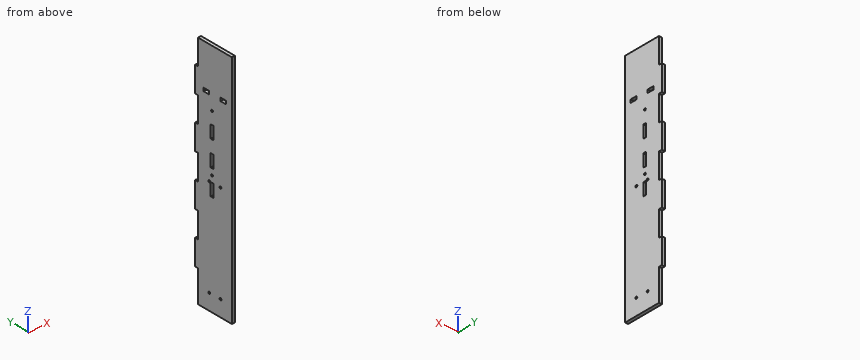
```python
from build123d import *

# Parameters (mm, degrees)
SKETCH1_W           = 6.35
SKETCH1_H           = 76.2
BOSS_EXTRUDE1_DEPTH = 457.2
SKETCH2_W           = 6.35
SKETCH2_H           = 50.8
BOSS_EXTRUDE2_DEPTH = 6.35
SKETCH3_W           = 6.35
SKETCH3_H           = 12.7
CUT_EXTRUDE1_DEPTH  = 460.399570091
SKETCH7_R           = 2.0955
CUT_EXTRUDE2_DEPTH  = 460.399570091
SKETCH9_R           = 2.0955
SKETCH9_W           = 25.4
SKETCH9_H           = 6.35
CUT_EXTRUDE3_DEPTH  = 6.35
SKETCH11_W          = 6.35
SKETCH11_H          = 76.2
BOSS_EXTRUDE5_DEPTH = 12.7


with BuildPart() as part:
    # Sketch1 → Boss-Extrude1 (new body)
    with BuildSketch(Plane.XY):
        with Locations((-41.275, 0)):
            Rectangle(SKETCH1_W, SKETCH1_H)
    extrude(amount=-BOSS_EXTRUDE1_DEPTH)

    # Sketch2 → Boss-Extrude2 (add)
    with BuildSketch(Plane(origin=(0, 38.1, 0), x_dir=(1, 0, 0), z_dir=(0, 1, 0))):
        with Locations((-41.275, 381)):
            Rectangle(SKETCH2_W, SKETCH2_H)
        with Locations((-41.275, 279.4)):
            Rectangle(SKETCH2_W, SKETCH2_H)
        with Locations((-41.275, 177.8)):
            Rectangle(SKETCH2_W, SKETCH2_H)
        with Locations((-41.275, 76.2)):
            Rectangle(SKETCH2_W, SKETCH2_H)
    extrude(amount=BOSS_EXTRUDE2_DEPTH)

    # Sketch3 → Cut-Extrude1 (cut, through all)
    with BuildSketch(Plane(origin=(-38.1, 0, 0), x_dir=(0, 0, -1), z_dir=(1, 0, 0))):
        with Locations((85.725, 19.05)):
            Rectangle(SKETCH3_W, SKETCH3_H)
        with Locations((85.725, -19.05)):
            Rectangle(SKETCH3_W, SKETCH3_H)
    extrude(amount=-CUT_EXTRUDE1_DEPTH, mode=Mode.SUBTRACT)

    # Sketch7 → Cut-Extrude2 (cut, through all)
    with BuildSketch(Plane.ZY.offset(44.45)):
        with Locations((-241.3, -12.7)):
            Circle(SKETCH7_R)
        with Locations((-241.3, 12.7)):
            Circle(SKETCH7_R)
        with Locations((-437.8325, -12.7)):
            Circle(SKETCH7_R)
        with Locations((-437.8325, 12.7)):
            Circle(SKETCH7_R)
    extrude(amount=-CUT_EXTRUDE2_DEPTH, mode=Mode.SUBTRACT)

    # Sketch9 → Cut-Extrude3 (cut)
    with BuildSketch(Plane.ZY.offset(44.45)):
        with Locations((-114.880216651, 6.35)):
            Circle(SKETCH9_R)
        with Locations((-228.517018256, 6.35)):
            Circle(SKETCH9_R)
        with Locations((-254, 6.35)):
            Rectangle(SKETCH9_W, SKETCH9_H)
        with Locations((-203.2, 6.35)):
            Rectangle(SKETCH9_W, SKETCH9_H)
        with Locations((-152.4, 6.35)):
            Rectangle(SKETCH9_W, SKETCH9_H)
    extrude(amount=-CUT_EXTRUDE3_DEPTH, mode=Mode.SUBTRACT)

    # Sketch11 → Boss-Extrude5 (add)
    with BuildSketch(Plane(origin=(0, 0, -457.2), x_dir=(-1, 0, 0), z_dir=(0, 0, -1))):
        with Locations((41.275, 0)):
            Rectangle(SKETCH11_W, SKETCH11_H)
    extrude(amount=BOSS_EXTRUDE5_DEPTH)


solid = part.part
```
Verification items for the finished model (mm, model axes). Round coordinates to 2 decimals unless told otherwise and drop trailing zeros.
1. Scan lines: L1, parallel to Y at x = -38.25, z = -162 (3 decimals); L2, parallel to Y at x = -40.5, z = -204 (3 decimals); L3, parallel to Z at x = -40.25, y = -21. Record each from-to range of solid material in increasing order.
2. Section check A-A on x = -40.25. State how many separate pieces and enclosed holes the cut face has, plus the area to 3 significant figures.
3. Gauge pin test, flat ends, axial feed: P1, Ø3, axis at x = -40, z = -25.5, coming from the +Y side; P2, Ø3, axis at x = -41.5, y = 42.5, coming from the -Z side. Record the tip position at first contact, or that the pin passes through.
Answer:
1. L1: y = -38.1 to 3.175, 9.525 to 44.45
1. L2: y = -38.1 to 3.175, 9.525 to 38.1
1. L3: z = -469.9 to -88.9, -82.55 to 0
2. separate pieces: 1
2. enclosed holes: 11
2. area: 36,400 mm2
3. P1: stops at y = 38.1
3. P2: stops at z = -406.4
